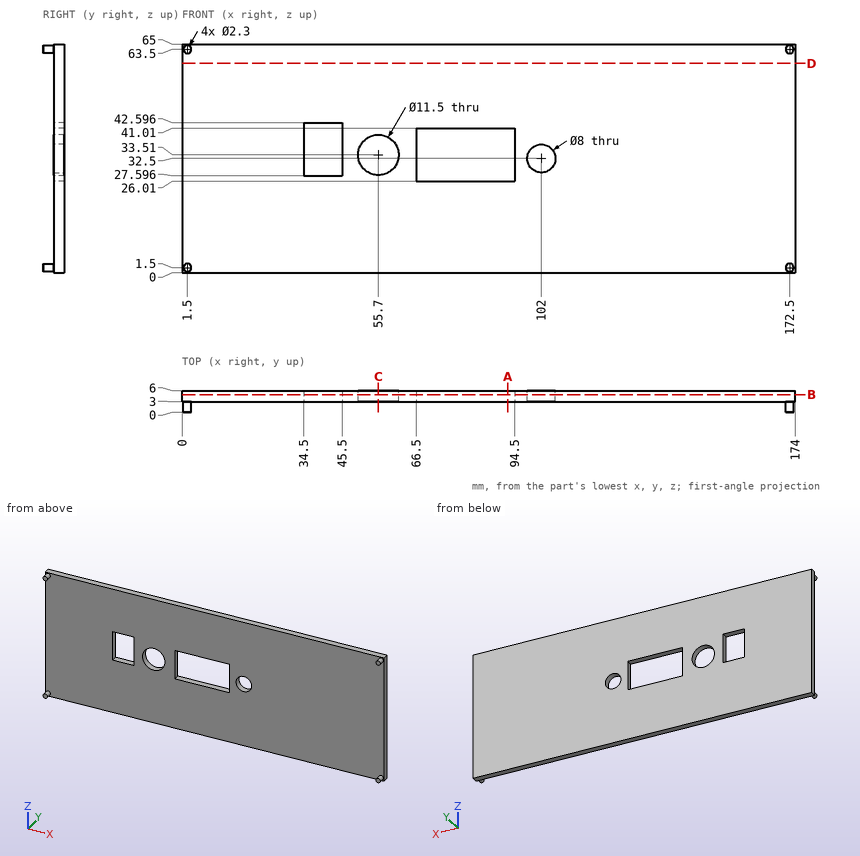
Check sheet for the drawn part. Datum: minimum x, y, z corner. Units: mm. Coordinates: 2 decimals unless noted, no trailing zeros. Order: outer loops, then holes, each group sorted by start corner. A loop starts at its lowest first (then second) coordinate and runs counter-clockwise, first axis right, second up. Notation, with made-up numbers: (-25.5, 7.25) - (6.5, 7.25) arc R21 cw to (6.5, 17.25) - close; hole circle Ø5 at (77, 56). An arc over 180 degrees is marked (long way). Return JSON: item names as keys, results as strings.
(1) Section check D-D, the plane z = 59.5. Record the cut outline in (x, y).
Filled sheet:
{"outline": "(0, 3) - (174, 3) - (174, 6) - (0, 6) - close"}
(2) Section check A-A, the plane x = 92.5. Record the cut outline in (y, z).
Filled sheet:
{"outline": "(3, 0) - (6, 0) - (6, 26.01) - (3, 26.01) - close; (3, 41.01) - (6, 41.01) - (6, 65) - (3, 65) - close"}
(3) Section check B-B, the plane y = 4.95. Record the cut outline in (x, z), and give its area (3 significant figures).
Filled sheet:
{"outline": "(0, 0) - (174, 0) - (174, 65) - (0, 65) - close; hole (34.5, 27.6) - (45.5, 27.6) - (45.5, 42.6) - (34.5, 42.6) - close; hole circle Ø11.5 at (55.7, 33.51); hole (66.5, 26.01) - (94.5, 26.01) - (94.5, 41.01) - (66.5, 41.01) - close; hole circle Ø8 at (102, 32.5)", "area": "10,600 mm^2"}
(4) Thickness scan on line 1 along X through (y, z) = (3.55, 40); line 2 along X through (y, z) = (4.85, 31.5); line 3 along Z through (x, y) = (76, 3.85). Record the ranges inside material, lowest first.
Filled sheet:
{"line 1": "x = 0 to 34.5, 45.5 to 66.5, 94.5 to 174", "line 2": "x = 0 to 34.5, 45.5 to 50.31, 61.09 to 66.5, 94.5 to 98.13, 105.87 to 174", "line 3": "z = 0 to 26.01, 41.01 to 65"}
(5) Go/stop test with flat-tipped pins: pin 1 (4 mm diameter, centred on x = 105, z = 10, fed in from -Y); pin 2 (9 mm diameter, centred on x = 55.7, z = 33.51, fed in from -Y); pin 3 (0.9 mm diameter, centred on y = 5, z = 34, fed in from -X). Record where each tip stops, or that it passes through.
Filled sheet:
{"pin 1": "stops at y = 3", "pin 2": "passes through", "pin 3": "stops at x = 0"}
(6) Section check C-C, the plane x = 55.7. Record the cut outline in (y, z).
Filled sheet:
{"outline": "(3, 0) - (6, 0) - (6, 27.76) - (3, 27.76) - close; (3, 39.26) - (6, 39.26) - (6, 65) - (3, 65) - close"}
